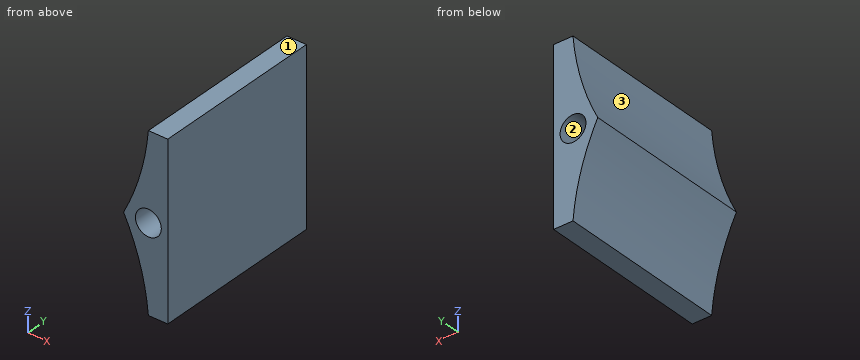
from build123d import *

# Parameters (mm, degrees)
SKETCH1_R           = 3
BOSS_EXTRUDE1_DEPTH = 40


with BuildPart() as part:
    # Sketch1 → Boss-Extrude1 (new body)
    with BuildSketch(Plane(origin=(0, 0, 0), x_dir=(1, 0, 0), z_dir=(0, 1, 0))):
        with BuildLine():
            Line((0, 20), (4.5, 20))
            Line((4.5, 20), (4.5, -20))
            Line((4.5, -20), (0, -20))
            ThreePointArc((0, -20), (-1.898782269, -9.719444247), (-5.749445099, 0))
            ThreePointArc((-5.749445099, 0), (-1.898782269, 9.719444247), (0, 20))
        make_face()
        with Locations(Location((0, 0, 0), (0, 0, 270))):
            Circle(SKETCH1_R, mode=Mode.SUBTRACT)
    extrude(amount=BOSS_EXTRUDE1_DEPTH)


solid = part.part
The listing builds one solid part. Answer for the finished solid, in the listing's coordinates (mm). Face numbers are marked on the shaded views. Round coordinates to 2 decimals unless told otherwise and drop trailing zeros. Order: outer loops, then holes, each group sorted by start corner. A loop starts at its lowest first (then second) coordinate and runs counter-clockwise, first axis right, second up. Notation, with made-up numbers: M 57,16.5 L 88,16.5 A14 cw 88,39.5 Z; hole C 54.25,33 d3. An arc over 180 degrees is marked long. Answer in a Markdown table with one row per item. Add a question column.
1) The part is cut by section A-A on y = 8.5. Determine the outline of the cut face in (x, z).
2) Determine the mould class of the marked faces 1, 2 and 3 for opening direction X: pulls with the +X half, pulls with the -X half, needs draft (parallel to the pull), parting line crosses it, or undercut.
3) Consider line 1 along X through (y, z) = (13.5, 2.5); line 2 along Z through (x, y) = (2, 21); line 3 along Z through (x, y) = (2.75, 31). Determine where each line is inside the solid, lowest interval first. Write a range as from..to.
4) The part is cut by section B-B on z = -0.5. Determine the outline of the cut face in (x, y).
5) The part is cut by section D-D on x = -4. Determine the outline of the cut face in (y, z), plus the area to 3 significant figures.
6) The part is cut by section C-C on z = 16. Determine the outline of the cut face in (x, y).
7) Flat-ended cylindrical pins translate along their axes: pin 1 Ø6 at (y, z) = (25.5, -2) entering from -X; pin 2 Ø3 at (y, z) = (25, -10.5) entering from -X. Find the tip coordinate at first contact, or state that the pin passes through.
Findings below:
| question | item | result |
|---|---|---|
| 1 | outline | M -5.75,0 A53.82 cw 0,-20 L 4.5,-20 L 4.5,20 L 0,20 A53.82 cw Z; hole C 0,0 d6 |
| 2 | face 1 | needs draft |
| 2 | face 2 | undercut |
| 2 | face 3 | pulls with the -X half |
| 3 | line 1 | x = -4.55..-1.66, 1.66..4.5 |
| 3 | line 2 | z = -20..-2.24, 2.24..20 |
| 3 | line 3 | z = -20..-1.2, 1.2..20 |
| 4 | outline | M -5.5,0 L -2.96,0 L -2.96,40 L -5.5,40 Z; M 2.96,0 L 4.5,0 L 4.5,40 L 2.96,40 Z |
| 5 | outline | M 0,-3.75 L 40,-3.75 L 40,3.75 L 0,3.75 Z |
| 5 | area | 300 mm² |
| 6 | outline | M -0.49,0 L 4.5,0 L 4.5,40 L -0.49,40 Z |
| 7 | pin 1 | stops at x = -5.75 |
| 7 | pin 2 | stops at x = -2.11 |
